Source: three-view drawing plus pictorial views. Frame: mm from the lowest corner of the part. Give positions to 0.01 mm unless a question says otherwise; leave off trailing zeros. Loops run counter-clockwise (first coordinate to the right, second up) from the corner with the lowest first, then second, coordinate; pieces in that order, holes last. Notation, with made-up numbers: (35, 41.25) - (79, 41.25) arc R22 cw to (79, 64.25) - close; hole circle Ø6 at (23.5, 89.5). An arc over 180 degrees is marked (long way). Answer as a JSON object with one key per item and string values. Group by question number.
(1) Section query C-C (y = 5.75). Return loops of the section in (x, z).
(2) Section query D-D (x = 17.5). Return loops of the section in (y, z), plus the area to 3 significant figures.
(3) Section query B-B (x = 88.9). Return loops of the section in (y, z).
(4) Material intervals for L1, parallel to Z at x = 93, y = 8.5; L2, parallel to Z at x = 101, y = 3.75; L3, parallel to X at y = 4.25, z = 114, sorted ascending.
(5) Section query A-A (z = 88.9). Return loops of the section in (x, y), plus the area to 3 significant figures.
(6) Pin query (flat end, axial travel): P1, Ø4, axis at x = 48.5, y = 2.5, coming from the -Z side; P2, Ø3, axis at x = 100, y = 6.5, coming from the -Z side; P3, Ø3, axis at y = 8, z = 21, coming from the +X side; P4, Ø4, axis at x = 54.5, z = 59.5, coming from the -Y side. Return the tip coordinate at first contact, or that it passes through.
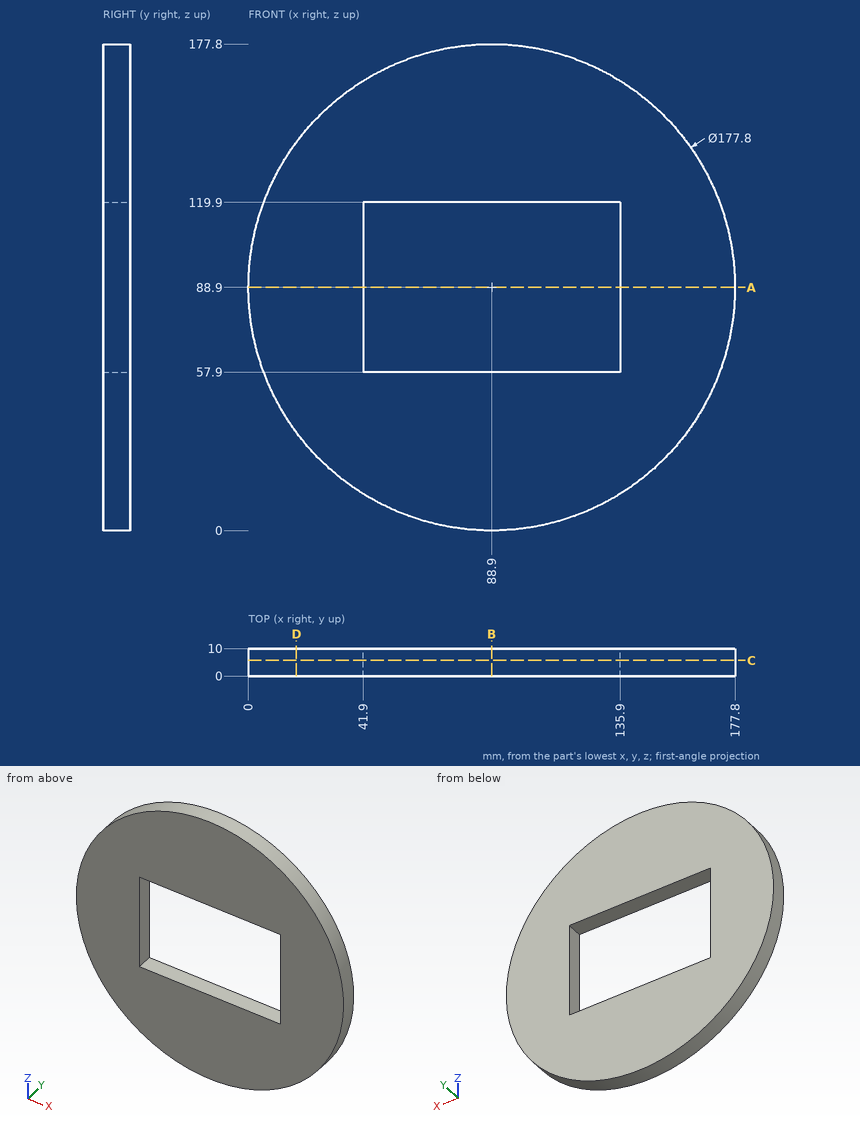
Recorded:
{
 "1": {"outline": "circle Ø177.8 at (88.9, 88.9); hole (41.9, 57.9) - (135.9, 57.9) - (135.9, 119.9) - (41.9, 119.9) - close"},
 "2": {"outline": "(0, 35.94) - (10, 35.94) - (10, 141.86) - (0, 141.86) - close", "area": "1,060 mm^2"},
 "3": {"outline": "(0, 0) - (10, 0) - (10, 57.9) - (0, 57.9) - close; (0, 119.9) - (10, 119.9) - (10, 177.8) - (0, 177.8) - close"},
 "4": {"L1": "z = 0.09 to 57.9, 119.9 to 177.71", "L2": "z = 0.83 to 57.9, 119.9 to 176.97", "L3": "x = 3.62 to 41.9, 135.9 to 174.18"},
 "5": {"outline": "(0, 0) - (41.9, 0) - (41.9, 10) - (0, 10) - close; (135.9, 0) - (177.8, 0) - (177.8, 10) - (135.9, 10) - close", "area": "838 mm^2"},
 "6": {"P1": "stops at z = 8.72", "P2": "stops at z = 0.52", "P3": "stops at x = 148.01", "P4": "stops at y = 0"}
}
